from build123d import *

# Parameters (mm, degrees)
SKETCH1_R                  = 10.15
MAIN_DEPTH                 = 45
SKETCH3_R                  = 16.25
MOTOREDUCTORMAINHOLE_DEPTH = 40
SKETCH2_R                  = 1.25
FIXHOLEMOTORS_DEPTH        = 10
HOLECIRCULARPATTERN_COUNT  = 4
SKETCH5_R                  = 3.25
HEADSCREWHOLE_DEPTH        = 2
SKETCH4_W                  = 50
SKETCH4_H                  = 35
HORIZONTALCUT_DEPTH        = 40
FILLET3_R                  = 15
SKETCH7_W                  = 50
SKETCH7_H                  = 2.9
MAKERBEAMRAIL_DEPTH        = 1
LPATTERN1_COUNT            = 4
LPATTERN1_PITCH            = 10
SKETCH6_R                  = 1.35
FIXTOPLATEHOLE_DEPTH       = 45.0000001
SKETCH9_R                  = 4.25
CUT_EXTRUDE2_DEPTH         = 36.0000001


with BuildPart() as part:
    # Sketch1 → Main (new body)
    with BuildSketch(Plane.XY):
        with BuildLine():
            Line((-25, -18), (-25, 0))
            ThreePointArc((-25, 0), (0, 25), (25, 0))
            Line((25, 0), (25, -18))
            Line((25, -18), (-25, -18))
        make_face()
        Circle(SKETCH1_R, mode=Mode.SUBTRACT)
    extrude(amount=MAIN_DEPTH)

    # Sketch3 → MotoReductorMainHole (cut)
    with BuildSketch(Plane.XY):
        Circle(SKETCH3_R)
    extrude(amount=MOTOREDUCTORMAINHOLE_DEPTH, mode=Mode.SUBTRACT)

    # Sketch2 → FixHoleMotors (cut)
    with BuildSketch(Plane.XY.offset(45)):
        with Locations((0, 13)):
            Circle(SKETCH2_R)
    fixholemotors = extrude(amount=-FIXHOLEMOTORS_DEPTH, mode=Mode.SUBTRACT)

    # HoleCircularPattern: FixHoleMotors ×4 about axis
    holecircularpattern_axis = Axis((0, 0, 0), (0, 0, 1))
    for i in range(1, HOLECIRCULARPATTERN_COUNT):
        add(fixholemotors.rotate(holecircularpattern_axis, i * 360 / HOLECIRCULARPATTERN_COUNT), mode=Mode.SUBTRACT)

    # Sketch5 → HeadScrewHole (cut)
    with BuildSketch(Plane.XY.offset(45)):
        with Locations((0, 13)):
            Circle(SKETCH5_R)
        with Locations((13, 0)):
            Circle(SKETCH5_R)
        with Locations((0, -13)):
            Circle(SKETCH5_R)
        with Locations((-13, 0)):
            Circle(SKETCH5_R)
    extrude(amount=-HEADSCREWHOLE_DEPTH, mode=Mode.SUBTRACT)

    # Sketch4 → HorizontalCut (cut)
    with BuildSketch(Plane(origin=(0, 0, 0), x_dir=(-1, 0, 0), z_dir=(0, 0, -1))):
        with Locations((0, 7.5)):
            Rectangle(SKETCH4_W, SKETCH4_H)
    extrude(amount=-HORIZONTALCUT_DEPTH, mode=Mode.SUBTRACT)

    # Fillet3
    fillet3_edges = [part.edges().sort_by_distance(p)[0] for p in [
        (-18.904344229, -10, 40),
        (18.904344229, -10, 40),
    ]]
    fillet(fillet3_edges, radius=FILLET3_R)

    # Sketch7 → MakerBeamRail (add)
    with BuildSketch(Plane(origin=(0, -18, 0), x_dir=(-1, 0, 0), z_dir=(0, -1, 0))):
        with Locations((0, -35)):
            Rectangle(SKETCH7_W, SKETCH7_H)
    makerbeamrail = extrude(amount=MAKERBEAMRAIL_DEPTH)

    # LPattern1: MakerBeamRail ×4
    with Locations(*[(0, 0, -i * LPATTERN1_PITCH) for i in range(1, LPATTERN1_COUNT)]):
        add(makerbeamrail)

    # Sketch6 → FixToPlateHole (cut, through all)
    with BuildSketch(Plane(origin=(0, -19, 0), x_dir=(-1, 0, 0), z_dir=(0, -1, 0))):
        with Locations((20, -35)):
            Circle(SKETCH6_R)
        with Locations((20, -15)):
            Circle(SKETCH6_R)
        with Locations((20, -25)):
            Circle(SKETCH6_R)
        with Locations((20, -5)):
            Circle(SKETCH6_R)
    fixtoplatehole = extrude(amount=-FIXTOPLATEHOLE_DEPTH, mode=Mode.SUBTRACT)

    # Sketch9 → Cut-Extrude2 (cut, through all)
    with BuildSketch(Plane(origin=(0, -10, 0), x_dir=(1, 0, 0), z_dir=(0, 1, 0))):
        with Locations((-20, -35)):
            Circle(SKETCH9_R)
    cut_extrude2 = extrude(amount=CUT_EXTRUDE2_DEPTH, mode=Mode.SUBTRACT)

    # Mirror1: FixToPlateHole, Cut-Extrude2 across plane
    add(fixtoplatehole.mirror(Plane(origin=(0, 0, 0), x_dir=(0, 0, 1), z_dir=(1, 0, 0))), mode=Mode.SUBTRACT)
    add(cut_extrude2.mirror(Plane(origin=(0, 0, 0), x_dir=(0, 0, 1), z_dir=(1, 0, 0))), mode=Mode.SUBTRACT)


solid = part.part
Build history of the part. All positions in model axes, mm. A direction names the side the tool comes from. Give positions to 0.01 mm unless a question says otherwise; leave off trailing zeros. Write each loop counter-clockwise with the first axis right and the second up, starting at its lowest first coordinate (ties: lowest second). Pieces come first, ordered by that corner, then holes. Notation, with made-up numbers: (19, 46.5) - (53, 46.5) arc R30 cw to (53, 85.5) - close; hole circle Ø3 at (55.25, 37). An arc over 180 degrees is marked (long way). Use one line per item in the form item = value. Start each with the question number.
1. Drop flat-ended pins along their axis: pin 1 Ø11 at (x, z) = (20, 35) entering from -Y; pin 2 Ø4 at (x, z) = (7, 26.5) entering from +Y; pin 3 Ø0.8 at (x, y) = (0.5, -18.5) entering from -Z; pin 4 Ø3 at (x, y) = (-20, 17) entering from -Z. Give the stop position or say it passes through.
2. Band-saw the part on D-D on z = 18. Write the cut outline in (x, y), plus the area to 3 significant figures.
3. 3-axis set-ups, long thin cutter, end or side, ignore diameter. For faces 1 (the face through (0, -18, 30)), 2 (the face through (1.4, 13.2, 43)), 3 (the face through (20.92, -6.06, 39.15)), 4 (the face through (0, -18, 2)): which of +Z, -Z, +X, -X, +Y, -Y reach the whole face in a straight line?
4. Probe line 1 (Y direction, x = 0, z = 41.2); line 2 (Z direction, x = 20, y = -13.75); line 3 (Y direction, x = 0, z = 44.3). List the from-to ranges inside material, lowest first. Write a range as [from, to].
5. Band-saw the part on A-A on y = -13. Count the separate pieces of the cut face and the enclosed holes in it, plus the area to 3 significant figures.
6. Two-plate mould, pull along Y, no slides. Class faces 5 (the face through (0, -18, 20)), 6 (the face through (6, 9, 45)), 7 (the face through (14.24, 0.16, 41.52)): released by +Y, released by -Y, zero draft, split by the parting line, or undercut.
7. Band-saw the part on C-C on z = 35. Write the cut outline in (x, y).
8. Band-saw the part on B-B on x = 7. Write the cut outline in (y, z) (3 decimals).
Conclusion:
q1.pin_1 = -19
q1.pin_2 = -13.53
q1.pin_3 = 3.55
q1.pin_4 = 40
q2.outline = (-25, -18) - (25, -18) - (25, -10) - (12.81, -10) arc R16.25 cw to (-12.81, -10) - (-25, -10) - close
q2.area = 288 mm²
q3.face_1 = +X, -X, -Y
q3.face_2 = +Z
q3.face_3 = +Y
q3.face_4 = -Z, +X, -X, -Y
q4.line_1 = [-18, -14.25], [-11.75, -10.15], [10.15, 11.75], [14.25, 25]
q4.line_2 = [0, 3.65], [6.35, 13.65], [16.35, 23.65], [26.35, 33.65], [36.35, 45]
q4.line_3 = [-18, -16.25], [16.25, 25]
q5.separate_pieces = 2
q5.enclosed_holes = 8
q5.area = 1,400 mm²
q6.face_5 = released by -Y
q6.face_6 = zero draft
q6.face_7 = undercut
q7.outline = (-25, -19) - (-21.35, -19) - (-21.35, -10) - (-24.25, -10) - (-24.25, -6.18) - (-25, -6.18) - close; (-18.65, -19) - (18.65, -19) - (18.65, -10) - (15.75, -10) - (15.75, -6.18) - (15.03, -6.18) arc R16.25 cw to (-15.03, -6.18) - (-15.75, -6.18) - (-15.75, -10) - (-18.65, -10) - close; (21.35, -19) - (25, -19) - (25, -6.18) - (24.25, -6.18) - (24.25, -10) - (21.35, -10) - close
q8.outline = (-19, 3.55) - (-18, 3.55) - (-18, 0) - (-14.665, 0) - (-14.665, 40) - (-7.35, 40) - (-7.35, 45) - (-18, 45) - (-18, 36.45) - (-19, 36.45) - (-19, 33.55) - (-18, 33.55) - (-18, 26.45) - (-19, 26.45) - (-19, 23.55) - (-18, 23.55) - (-18, 16.45) - (-19, 16.45) - (-19, 13.55) - (-18, 13.55) - (-18, 6.45) - (-19, 6.45) - close; (7.35, 40) - (24, 40) - (24, 45) - (7.35, 45) - close
